from build123d import *

# Parameters (mm, degrees)
SKETCH1_W           = 70.866
SKETCH1_H           = 46.99
BOSS_EXTRUDE1_DEPTH = 8.636
SKETCH2_W           = 63.246
SKETCH2_H           = 39.37
CUT_EXTRUDE1_DEPTH  = 7.366
FILLET2_R           = 7.62
FILLET3_R           = 3.81


with BuildPart() as part:
    # Sketch1 → Boss-Extrude1 (new body)
    with BuildSketch(Plane(origin=(0, 0, 0), x_dir=(1, 0, 0), z_dir=(0, 1, 0))):
        with Locations((35.433, 23.495)):
            Rectangle(SKETCH1_W, SKETCH1_H)
    extrude(amount=BOSS_EXTRUDE1_DEPTH)

    # Sketch2 → Cut-Extrude1 (cut)
    with BuildSketch(Plane(origin=(0, 8.636, 0), x_dir=(1, 0, 0), z_dir=(0, 1, 0))):
        with Locations((35.433, 23.495)):
            Rectangle(SKETCH2_W, SKETCH2_H)
    extrude(amount=-CUT_EXTRUDE1_DEPTH, mode=Mode.SUBTRACT)

    # Fillet2
    fillet2_edges = [part.edges().sort_by_distance(p)[0] for p in [
        (0, 4.318, -46.99),
        (70.866, 4.318, -46.99),
        (70.866, 4.318, 0),
        (0, 4.318, 0),
    ]]
    fillet(fillet2_edges, radius=FILLET2_R)

    # Fillet3
    fillet3_edges = [part.edges().sort_by_distance(p)[0] for p in [
        (35.433, 0, -46.99),
        (0, 0, -23.495),
        (70.866, 0, -23.495),
        (35.433, 0, 0),
        (2.231846327, 0, -44.758153673),
        (2.231846327, 0, -2.231846327),
        (68.634153673, 0, -2.231846327),
        (68.634153673, 0, -44.758153673),
    ]]
    fillet(fillet3_edges, radius=FILLET3_R)


solid = part.part
The listing builds one solid part. Answer for the finished solid, in the listing's coordinates (mm). A direction names the side the tool comes from. Coordinates: 2 decimals unless noted, no trailing zeros. Order: outer loops, then holes, each group sorted by start corner. A loop starts at its lowest first (then second) coordinate and runs counter-clockwise, first axis right, second up. Notation, with made-up numbers: (-40, 74.25) -> (-3, 74.25) arc R23 ccw to (-3, 101.25) -> close; hole circle Ø5 at (84.5, 36). An arc over 180 degrees is marked (long way). Answer in a Markdown table with one row per item. Add a question column.
Item 1: Determine the mould class of faces 3 (the face through (35.822, 1.086, -45.844)), 4 (the face through (67.056, 5, -23)), 5 (the face through (0, 6, -23)) for opening direction Z: +Z half, -Z half, draft (parallel to the pull), parting line (faces both ways), or undercut.
Item 2: Find the intervals of material crossed by L1, parallel to X at y = 6.5, z = -31; L2, parallel to Z at x = 37, y = 7.5; L3, parallel to Y at x = 15, z = -39.5, in increasing order. Write a range as from..to.
Item 3: Find section B-B (x = 18.5). Write down the section's boundary in (y, z), then the cut area to 3 significant figures.
Item 4: Find section A-A (y = 6). Write down the section's boundary in (x, z), then the cut area to 3 significant figures.
Item 5: Which of the six approach directions +Z, -Z, +X, -X, +Y, -Y give full straight-line access (tool end or side, diameter ignored) to faces 1 (the face through (69.72, 1.086, -23.273)), 2 (the face through (35, 1.27, -24))?
Item 6: Each of these flat-tipped pins is pushed along its axis until it touches: P1, Ø1.5, axis at y = 1.5, z = -18.5, coming from the +X side; P2, Ø5, axis at y = 2, z = -12, coming from the -X side; P3, Ø1, axis at x = 19.5, z = -21, coming from the +Y side. Where does it stop, or does it pass through?
Item 7: Find section C-C (z = -30). Write down the section's boundary in (x, y).
Result set:
| question | item | result |
|---|---|---|
| 1 | face 3 | -Z half |
| 1 | face 4 | undercut |
| 1 | face 5 | draft |
| 2 | L1 | x = 0..3.81, 67.06..70.87 |
| 2 | L2 | z = -46.99..-43.18, -3.81..0 |
| 2 | L3 | y = 0..1.27 |
| 3 | outline | (0, -43.18) arc R3.81 ccw to (3.81, -46.99) -> (8.64, -46.99) -> (8.64, -43.18) -> (1.27, -43.18) -> (1.27, -3.81) -> (8.64, -3.81) -> (8.64, 0) -> (3.81, 0) arc R3.81 ccw to (0, -3.81) -> close |
| 3 | area | 110 mm² |
| 4 | outline | (0, -39.37) arc R7.62 ccw to (7.62, -46.99) -> (63.25, -46.99) arc R7.62 ccw to (70.87, -39.37) -> (70.87, -7.62) arc R7.62 ccw to (63.25, 0) -> (7.62, 0) arc R7.62 ccw to (0, -7.62) -> close; hole (3.81, -43.18) -> (67.06, -43.18) -> (67.06, -3.81) -> (3.81, -3.81) -> close |
| 4 | area | 790 mm² |
| 5 | face 1 | +Z, -Z, +X, -Y |
| 5 | face 2 | +Y |
| 6 | P1 | stops at x = 70.53 |
| 6 | P2 | stops at x = 0 |
| 6 | P3 | stops at y = 1.27 |
| 7 | outline | (0, 3.81) arc R3.81 ccw to (3.81, 0) -> (67.06, 0) arc R3.81 ccw to (70.87, 3.81) -> (70.87, 8.64) -> (67.06, 8.64) -> (67.06, 1.27) -> (3.81, 1.27) -> (3.81, 8.64) -> (0, 8.64) -> close |
